The model under review builds one solid part; all positions refer to its coordinate system, in mm. A direction names the side the tool comes from. Coordinates: 2 decimals unless noted, no trailing zeros. Write each loop counter-clockwise with the first axis right and the second up, starting at its lowest first coordinate (ties: lowest second). Pieces come first, ordered by that corner, then holes.
1) Machinability: for faces 4 (the flat face through (-98, -740, 0)), 5 (the flat face through (-98, -740, 4)), which of the approach directions +Z, -Z, +X, -X, +Y, -Y give a long, thin tool a straight path to every point of the face, cutting with its end or side? Answer none if there is none.
2) Add section D-D, the plane x = -30.5. State the section outline as (y, z) points, then the cut area to 3 significant figures.
3) For line 1 (Z direction, x = -90.5, y = -176.5); line 2 (X direction, y = -159, z = 2), list the stretches that pass through material, from the lowest coordinate up.
4) Add section C-C, the plane z = 22.5. State the section outline as (x, y) points, then the cut area to 3 significant figures.
5) Mouldability with a two-part tool opening along Y and no side actions: class faces 1 (the flat face through (-53, 0, 3)), 2 (the flat face through (0, -740, 34)), 3 (the flat face through (-53, -1500, 3)) as released by +Y, released by -Y, zero draft, split by the parting line, or undercut.
6) For P1, Ø1.2, axis at y = -398.5, z = 1.5, coming from the -X side; P2, Ø8, axis at y = -633, z = 42, coming from the -X side, all flat-tipped, find the tip position at first contact; note any pin that passes through.
7) Add section B-B, the plane y = -1215. State the section outline as (x, z) points.
8) Add section A-A, the plane x = -117. State the section outline as (y, z) points, then the cut area to 3 significant figures.
Autodesk Inventor part; units mm, degrees
ref_plane "YZ Plane" through (0, 0, 0) normal (1, 0, 0) x (0, 1, 0)
ref_plane "XZ Plane" through (0, 0, 0) normal (0, 1, 0) x (-1, 0, 0)
ref_plane "XY Plane" through (0, 0, 0) normal (0, 0, 1) x (1, 0, 0)
sketch "Sketch1" plane through (0, 0, 0) normal (0, 0, 1) x (1, 0, 0)
  line L0 (0, 0) -> (-190.3129, 0)
  line L1 (-190.3129, 0) -> (-190.3129, -1500)
  line L2 (-190.3129, -1500) -> (0, -1500)
  line L3 (0, -1500) -> (0, 0)
  line L4 (-190.3129, -1400) -> (-66, -1400)
  line L5 (-66, -1400) -> (-66, -1395)
  line L6 (-66, -1395) -> (-190.3129, -1395)
  line L7 (-190.3129, -1395) -> (-190.3129, -1400)
  line L8 (-190.3129, -900) -> (-66, -900)
  line L9 (-66, -900) -> (-66, -895)
  line L10 (-66, -895) -> (-190.3129, -895)
  line L11 (-190.3129, -895) -> (-190.3129, -900)
  line L12 (-190.3129, -400) -> (-66, -400)
  line L13 (-66, -400) -> (-66, -395)
  line L14 (-66, -395) -> (-190.3129, -395)
  line L15 (-190.3129, -395) -> (-190.3129, -400)
  circle A0 centre (-190.3129, 0) radius 30
  circle A1 centre (-190.3129, -1500) radius 30
  point P0 (-190.3129, -395)
  point P1 (-190.3129, -400)
  point P2 (-190.3129, -1395)
  point P3 (-160.3129, 0)
  point P4 (-190.3129, -30)
  point P5 (-190.3129, -1470)
  point P6 (-160.3129, -1500)
  dimension "d0" = 1500
  dimension "d1" = 190.3129
  dimension "d2" = 5
  dimension "d4" = 100
  dimension "d7" = 500
  dimension "d23" = 66
  dimension "d24" = 60
extrude "Plate1" add sketch "Sketch1" along normal blind 4 contours L3 L2 A1 L1 L4 L5 L6 L8 L9 L10 L12 L13 L14 A0 L0
sketch "Sketch2" plane through (4, 0, 0) normal (-1, 0, 0) x (0, -1, 0)
  line L0 (1500, 0) -> (0, 0)
  line L1 (0, 0) -> (0, 60)
  line L2 (0, 60) -> (1500, 60)
  line L3 (1500, 60) -> (1500, 0)
edge flange "Flange1" height 60 angle 90 thickness 4 bend radius 4 thickness toward (-1, 0, 0) relief tear relief width 4 relief depth 2 edges at (0, -750, 4) wall of the first edge with corners at (4, -1500, 0) (4, 0, 0) (4, 0, 60) (4, -1500, 60)
bend "Bend1"
corner "Corner1"
chamfer "Corner Chamfer1" distance 3 angle 45 6 edges at (-190.3129, -1400, 2) (-190.3129, -1395, 2) (-190.3129, -900, 2) (-190.3129, -895, 2) (-190.3129, -395, 2) (-190.3129, -400, 2)
equation "\"d1\" = стрингер_глубина_1"
equation "\"d2\" = паз_под_стрингер_толщина"
equation "\"d23\" = паз_под_стрингер_глубина - Thickness"
equation "\"d24\" = 2 * радиус_выреза_под_сварку"
equation "\"d12\" = Thickness"
equation "\"d13\" = BendReliefWidth"
equation "\"d14\" = BendReliefDepth"
equation "\"d15\" = MinimumRemnant"
equation "\"d16\" = TransitionRadius"
equation "\"d17\" = ребро_усилителей"
equation "\"d19\" = BendRadius"
equation "\"d20\" = CornerReliefSize"
equation "\"d21\" = GapSize"
equation "\"d22\" = JacobiRadiusSize"
equation "\"BendRadius\" = Thickness"
equation "\"BendReliefWidth\" = Thickness"
equation "\"BendReliefDepth\" = 0.5 * Thickness"
equation "\"CornerReliefSize\" = 4 * Thickness"
equation "\"MinimumRemnant\" = 2 * Thickness"
equation "\"TransitionRadius\" = BendRadius"
equation "\"JacobiRadiusSize\" = BendRadius"
equation "\"GapSize\" = Thickness"
properties part number "01.3 GBK stringer 1" material "Steel"
Geometry results:
1. face 4: -Z, +X, -X, +Y, -Y
1. face 5: +Z, -X, +Y, -Y
2. outline: (-1500, 0) - (0, 0) - (0, 4) - (-1500, 4) - close
2. area: 6,000 mm2
3. line 1: z = 0 to 4
3. line 2: x = -190.31 to 1.29
4. outline: (0, -1500) - (4, -1500) - (4, 0) - (0, 0) - close
4. area: 6,000 mm2
5. face 1: released by +Y
5. face 2: zero draft
5. face 3: released by -Y
6. P1: stops at x = -66
6. P2: stops at x = 0
7. outline: (-190.31, 0) - (-4, 0) arc R8 ccw to (4, 8) - (4, 60) - (0, 60) - (0, 8) arc R4 cw to (-4, 4) - (-190.31, 4) - close
8. outline: (-1500, 0) - (-1400, 0) - (-1400, 4) - (-1500, 4) - close; (-1395, 0) - (-900, 0) - (-900, 4) - (-1395, 4) - close; (-895, 0) - (-400, 0) - (-400, 4) - (-895, 4) - close; (-395, 0) - (0, 0) - (0, 4) - (-395, 4) - close
8. area: 5,940 mm2
